```python
from build123d import *

# Parameters (mm, degrees)
SKETCH1_W               = 70
SKETCH1_H               = 40
SKETCH1_R               = 7.5
BOSS_EXTRUDE2_DEPTH     = 10
SKETCH2_R               = 10
CUT_EXTRUDE1_DEPTH      = 7
SKETCH3_W               = 10
SKETCH3_H               = 40
BOSS_EXTRUDE3_DEPTH     = 53
SKETCH5_W               = 30
SKETCH5_H               = 40
BOSS_EXTRUDE4_DEPTH     = 10
SKETCH7_R               = 2
CUT_EXTRUDE2_DEPTH      = 10
FILLET5_R               = 5
FILLET6_R               = 5
SKETCH10_W              = 70
SKETCH10_H              = 45
SKETCH10_R              = 10
BOSS_EXTRUDE9_DEPTH     = 10
CUT_EXTRUDE3_DEPTH      = 96.771597908
CUT_EXTRUDE3_DEPTH_BACK = 6
SKETCH11_R              = 19
FILLET7_R               = 10
FILLET8_R               = 10
FILLET9_R               = 5


with BuildPart() as part:
    # Sketch1 → Boss-Extrude2 (new body)
    with BuildSketch(Plane(origin=(0, 0, 0), x_dir=(1, 0, 0), z_dir=(0, 1, 0))):
        Rectangle(SKETCH1_W, SKETCH1_H)
        with Locations(Location((0, 0.222850833, 0), (0, 0, 270))):
            Circle(SKETCH1_R, mode=Mode.SUBTRACT)
    extrude(amount=BOSS_EXTRUDE2_DEPTH)

    # Sketch2 → Cut-Extrude1 (cut)
    with BuildSketch(Plane(origin=(0, 10, 0), x_dir=(1, 0, 0), z_dir=(0, 1, 0))):
        with Locations(Location((0, 0, 0), (0, 0, 270))):
            Circle(SKETCH2_R)
    extrude(amount=-CUT_EXTRUDE1_DEPTH, mode=Mode.SUBTRACT)

    # Sketch3 → Boss-Extrude3 (add)
    with BuildSketch(Plane.XZ):
        with Locations((-30, 0)):
            Rectangle(SKETCH3_W, SKETCH3_H)
    boss_extrude3 = extrude(amount=BOSS_EXTRUDE3_DEPTH)

    # Sketch5 → Boss-Extrude4 (add)
    with BuildSketch(Plane.XZ.offset(53)):
        with Locations((-40, 0)):
            Rectangle(SKETCH5_W, SKETCH5_H)
    boss_extrude4 = extrude(amount=-BOSS_EXTRUDE4_DEPTH)

    # Sketch7 → Cut-Extrude2 (cut)
    with BuildSketch(Plane.XZ.offset(53)):
        with Locations(Location((-47, 12, 0), (0, 0, 270))):
            Circle(SKETCH7_R)
        with Locations(Location((-47, -12, 0), (0, 0, 270))):
            Circle(SKETCH7_R)
    cut_extrude2 = extrude(amount=-CUT_EXTRUDE2_DEPTH, mode=Mode.SUBTRACT)

    # Fillet5
    fillet5_edges = [part.edges().sort_by_distance(p)[0] for p in [
        (-35, -43, 0),
    ]]
    fillet(fillet5_edges, radius=FILLET5_R)

    # Mirror10: Boss-Extrude3, Boss-Extrude4, Cut-Extrude2 across plane
    add(boss_extrude3.mirror(Plane(origin=(0, 0, 0), x_dir=(0, 0, 1), z_dir=(1, 0, 0))))
    add(boss_extrude4.mirror(Plane(origin=(0, 0, 0), x_dir=(0, 0, 1), z_dir=(1, 0, 0))))
    add(cut_extrude2.mirror(Plane(origin=(0, 0, 0), x_dir=(0, 0, 1), z_dir=(1, 0, 0))), mode=Mode.SUBTRACT)

    # Fillet6
    fillet6_edges = [part.edges().sort_by_distance(p)[0] for p in [
        (35, -43, 0),
    ]]
    fillet(fillet6_edges, radius=FILLET6_R)

    # Sketch10 → Boss-Extrude9 (add)
    with BuildSketch(Plane(origin=(0, 0, 0), x_dir=(1, 0, 0), z_dir=(0, 1, 0))):
        with Locations((-0.013568797, -35.277149167)):
            Rectangle(SKETCH10_W, SKETCH10_H)
        with Locations(Location((-0.013568797, -35.277149167, 0), (0, 0, 270))):
            Circle(SKETCH10_R, mode=Mode.SUBTRACT)
    extrude(amount=-BOSS_EXTRUDE9_DEPTH)

    # Sketch11 → Cut-Extrude3 (cut, two sides: drawn at the far end of the back side and taken through both)
    with BuildSketch(Plane(origin=(0, 0, 0), x_dir=(1, 0, 0), z_dir=(0, 1, 0)).offset(-CUT_EXTRUDE3_DEPTH_BACK)):
        with Locations(Location((-0.013568797, -35.277149167, 0), (0, 0, 126.480381765))):
            Circle(SKETCH11_R)
    extrude(amount=CUT_EXTRUDE3_DEPTH + CUT_EXTRUDE3_DEPTH_BACK, mode=Mode.SUBTRACT)

    # Fillet7
    # the kernel refuses this fillet: 10 mm, written as the material it adds along each edge
    with BuildSketch(Plane(origin=(-35, -10, 20), x_dir=(0, 0, 1), z_dir=(1, 0, 0))) as fillet7_piece_1:
        with BuildLine():
            CenterArc((FILLET7_R, FILLET7_R), FILLET7_R, 180, 90)
            Line((0, FILLET7_R), (0, 0))
            Line((0, 0), (FILLET7_R, 0))
        make_face()
    extrude(amount=10)
    with BuildSketch(Plane(origin=(25, -10, 20), x_dir=(0, -1, 0), z_dir=(1, 0, 0))) as fillet7_piece_2:
        with BuildLine():
            CenterArc((FILLET7_R, -FILLET7_R), FILLET7_R, 90, 90)
            Line((0, -FILLET7_R), (0, 0))
            Line((0, 0), (FILLET7_R, 0))
        make_face()
    extrude(amount=9.986431203)
    with BuildSketch(Plane(origin=(-13.717166125, 0, 20), x_dir=(0, 1, 0), z_dir=(1, 0, 0))) as fillet7_piece_3_section:
        with BuildLine():
            CenterArc((FILLET7_R, FILLET7_R), FILLET7_R, 180, 90)
            Line((0, FILLET7_R), (0, 0))
            Line((0, 0), (FILLET7_R, 0))
        make_face()
    fillet7_piece_3 = extrude(amount=48.703597328, mode=Mode.PRIVATE)
    fillet7_piece_3 = fillet7_piece_3 - Plane(origin=(-0.013568797, 3.73467358, 35.277149167), x_dir=(-0.5945475090531093, 0, -0.8040604824755057), z_dir=(0, -1, 0)) * Cylinder(19, 138, mode=Mode.PRIVATE)
    add(fillet7_piece_3)
    with BuildSketch(Plane(origin=(-35, 0, 20), x_dir=(0, 0, 1), z_dir=(1, 0, 0))) as fillet7_piece_4_section:
        with BuildLine():
            CenterArc((FILLET7_R, -FILLET7_R), FILLET7_R, 90, 90)
            Line((0, -FILLET7_R), (0, 0))
            Line((0, 0), (FILLET7_R, 0))
        make_face()
    fillet7_piece_4 = extrude(amount=48.690028531, mode=Mode.PRIVATE)
    fillet7_piece_4 = fillet7_piece_4 - Plane(origin=(-0.013568797, 2.378365403, 35.277149167), x_dir=(-0.5945475090531093, 0, -0.8040604824755057), z_dir=(0, -1, 0)) * Cylinder(19, 138, mode=Mode.PRIVATE)
    add(fillet7_piece_4)

    # Fillet8
    fillet8_edges = [part.edges().sort_by_distance(p)[0] for p in [
        (25, 0, -3.611425416),
        (-25, 0, -3.611425416),
        (-25, -10, 21.388574584),
        (25, -10, 21.388574584),
    ]]
    fillet(fillet8_edges, radius=FILLET8_R)

    # Fillet9
    fillet9_edges = [part.edges().sort_by_distance(p)[0] for p in [
        (0, 0, 12.777149167),
        (-22.071067812, -2.928932188, 12.777149167),
        (22.071067812, -2.928932188, 12.777149167),
        (25, -15, 12.777149167),
        (-25, -15, 12.777149167),
    ]]
    fillet(fillet9_edges, radius=FILLET9_R)


solid = part.part
```
Read the model definition and answer for the solid it produces. Units are mm, in the model's axes. A direction names the side the tool comes from. Give positions to 0.01 mm unless a question says otherwise; leave off trailing zeros. Write each loop counter-clockwise with the first axis right and the second up, starting at its lowest first coordinate (ties: lowest second). Pieces come first, ordered by that corner, then holes. Notation, with made-up numbers: (61, 57) - (109, 57) arc R24 cw to (109, 95) - close; hole circle Ø4 at (-33.5, 82.25). An arc over 180 degrees is marked (long way). Write item = value, one per line. Start each with the question number.
Item 1: Find the intervals of material crossed by probe 1 along X at (y, z) = (-48, 12); probe 2 along X at (y, z) = (-17, 4); probe 3 along Y at (x, z) = (-4, 53), in increasing order. Write a range as [from, to].
Item 2: The mould has two halves that part along X. Classify faces 5 (the flat face through (-33, -40, 20)), 6 (the flat face through (-35.014, -5, 36)), 7 (the flat face through (34.986, -5, 37)), 8 (the flat face through (0, -7, 12.777)): +X half, -X half, draft (parallel to the pull), parting line (faces both ways), or undercut.
Item 3: Find section A-A (x = -47). Give the vertices of the cut face in (y, z), then the cut area to 3 significant figures.
Item 4: Find section B-B (z = -12). Give the vertices of the cut face in (x, y).
Item 5: A tool of negligible diameter and unlimited length cuts with its end or side. For faces 1 (the cylindrical face through (21.99, -12.85, 19.04)), 2 (the flat face through (0, 0, -9)), 3 (the flat face through (-8, -10, 45)), 4 (the flat face through (2, -6, 24)), from which of +Z, -Z, +X, -X, +Y, -Y can it reach the whole face along a straight path? Write none if from no direction.
Item 6: Each of these flat-tipped pins is pushed along its axis until it touches: P1, Ø23, axis at x = -0.01, z = 35.28, coming from the -Y side; P2, Ø6.5, axis at x = 47, z = 12, coming from the -Y side; P3, Ø3, axis at x = 47, z = -12, coming from the +Y side; P4, Ø12, axis at x = 0, z = 43, coming from the +Y side. Where does it stop, or does it pass through?
Item 7: Find section D-D (z = 0). Give the vertices of the cut face in (x, y), then the cut area to 3 significant figures.
Response:
q1.probe_1 = [-55, -49], [-45, -25], [25, 45], [49, 55]
q1.probe_2 = [-35, -25], [25, 35]
q1.probe_3 = [-10, -6]
q2.face_5 = draft
q2.face_6 = -X half
q2.face_7 = +X half
q2.face_8 = undercut
q3.outline = (-53, -20) - (-43, -20) - (-43, -14) - (-53, -14) - close; (-53, -10) - (-43, -10) - (-43, 10) - (-53, 10) - close; (-53, 14) - (-43, 14) - (-43, 20) - (-53, 20) - close
q3.area = 320 mm²
q4.outline = (-55, -53) - (-49, -53) - (-49, -43) - (-55, -43) - close; (-45, -53) - (-25, -53) - (-25, -10) arc R10 cw to (-15, 0) - (15, 0) arc R10 cw to (25, -10) - (25, -53) - (45, -53) - (45, -43) - (40, -43) arc R5 cw to (35, -38) - (35, 10) - (-35, 10) - (-35, -38) arc R5 cw to (-40, -43) - (-45, -43) - close; (49, -53) - (55, -53) - (55, -43) - (49, -43) - close
q5.face_1 = +Z, -Z, -Y
q5.face_2 = -Z, -Y
q5.face_3 = +Z, -Y
q5.face_4 = +Y
q6.P1 = -10
q6.P2 = -53
q6.P3 = through
q6.P4 = -6
q7.outline = (-55, -53) - (-25, -53) - (-25, -10) arc R10 cw to (-15, 0) - (-7.5, 0) - (-7.5, 3) - (-10, 3) - (-10, 10) - (-35, 10) - (-35, -38) arc R5 cw to (-40, -43) - (-55, -43) - close; (7.5, 0) - (15, 0) arc R10 cw to (25, -10) - (25, -53) - (55, -53) - (55, -43) - (40, -43) arc R5 cw to (35, -38) - (35, 10) - (10, 10) - (10, 3) - (7.5, 3) - close
q7.area = 2,030 mm²
